Design review of the part built by this model. Coordinates are the model's own, in mm. Round coordinates to 2 decimals unless told otherwise and drop trailing zeros. Loops run counter-clockwise (first coordinate to the right, second up) from the corner with the lowest first, then second, coordinate; pieces in that order, holes last. Notation, with made-up numbers: (67, 76) - (109, 76) arc R23 cw to (109, 97) - close; hole circle Ø9 at (-24, 21). An arc over 180 degrees is marked (long way). Return JSON: item names as keys, results as strings. Group by question number.
(1) Clearance check with a flat-ended pin moving along its axis: pin 1 (12 mm diameter, centred on x = 83, z = 1, fed in from +Y). State where the tip first meets the part, or that it passes through.
(2) The part is to be moulded in two halves that separate along Z. For faces 1 (the cylindrical face through (-82.53, -25.04, 0.84)), 2 (the flat face through (-2, -23, -76.2)), 3 (the flat face through (27, -50.8, 1)), 4 (the cylindrical face through (44.47, -25.04, 0.84)), say which applies: pulls with the +Z half, pulls with the -Z half, needs draft (parallel to the pull), parting line crosses it, or undercut.
(3) We need section A-A, the plane z = 0. Write out the cut boundary in (x, y).
(4) We need section C-C, the plane x = 0. Write out the cut boundary in (y, z).
(5) We need section D-D, the plane x = 60. Write out the cut boundary in (y, z), and give its area (3 significant figures).
(6) Wall thickness on L1, parallel to Z at x = 0, y = -27.5; L2, parallel to Z at x = 106, y = -46; L3, parallel to Z at x = 61.5, y = -4.5: over which ranges is each line inside the solid? List them lowest first. Write a range as [from, to].
(7) We need section B-B, the plane y = -32. Write out the cut boundary in (x, z).
from build123d import *

# Parameters (mm, degrees)
F0_W     = 266.7
F0_H     = 152.4
F1_DEPTH = 50.8
F2_R     = 19.05
F3_DEPTH = 76.2
F4_R     = 19.05
F5_DEPTH = 50.8
F6_R     = 19.05
F7_DEPTH = 50.8
F8_R     = 5.08


with BuildPart() as f1:
    # F0 (on Front) → F1 (new body)
    with BuildSketch(Plane.XZ):
        Rectangle(F0_W, F0_H)
    extrude(amount=F1_DEPTH)

    # F2 (on face) → F3 (cut)
    with BuildSketch(Plane.XZ.offset(50.8)):
        Circle(F2_R)
    extrude(amount=-F3_DEPTH, mode=Mode.SUBTRACT)

    # F4 (on Front) → F5 (cut)
    with BuildSketch(Plane.XZ):
        with Locations((-63.5, 0)):
            Circle(F4_R)
    extrude(amount=F5_DEPTH, mode=Mode.SUBTRACT)

    # F6 (on Front) → F7 (cut)
    with BuildSketch(Plane.XZ):
        with Locations((63.5, 0)):
            Circle(F6_R)
    extrude(amount=F7_DEPTH, mode=Mode.SUBTRACT)

    # F8
    f8_edges = [f1.edges().sort_by_distance(p)[0] for p in [
        (0, -50.8, 76.2),
        (-133.35, -50.8, 0),
        (0, -50.8, -76.2),
        (133.35, -50.8, 0),
    ]]
    fillet(f8_edges, radius=F8_R)


solid = f1.part
Solutions:
{
 "1": {"pin 1": "y = 0"},
 "2": {"face 1": "undercut", "face 2": "pulls with the -Z half", "face 3": "needs draft", "face 4": "undercut"},
 "3": {"outline": "(-133.35, -45.72) arc R5.08 ccw to (-128.27, -50.8) - (-82.55, -50.8) - (-82.55, 0) - (-133.35, 0) - close; (-44.45, -50.8) - (-19.05, -50.8) - (-19.05, 0) - (-44.45, 0) - close; (19.05, -50.8) - (44.45, -50.8) - (44.45, 0) - (19.05, 0) - close; (82.55, -50.8) - (128.27, -50.8) arc R5.08 ccw to (133.35, -45.72) - (133.35, 0) - (82.55, 0) - close"},
 "4": {"outline": "(-50.8, -71.12) arc R5.08 ccw to (-45.72, -76.2) - (0, -76.2) - (0, -19.05) - (-50.8, -19.05) - close; (-50.8, 19.05) - (0, 19.05) - (0, 76.2) - (-45.72, 76.2) arc R5.08 ccw to (-50.8, 71.12) - close"},
 "5": {"outline": "(-50.8, -71.12) arc R5.08 ccw to (-45.72, -76.2) - (0, -76.2) - (0, -18.73) - (-50.8, -18.73) - close; (-50.8, 18.73) - (0, 18.73) - (0, 76.2) - (-45.72, 76.2) arc R5.08 ccw to (-50.8, 71.12) - close", "area": "5,830 mm^2"},
 "6": {"L1": "[-76.2, -19.05], [19.05, 76.2]", "L2": "[-76.19, 76.19]", "L3": "[-76.2, -18.94], [18.94, 76.2]"},
 "7": {"outline": "(-133.35, -76.2) - (133.35, -76.2) - (133.35, 76.2) - (-133.35, 76.2) - close; hole circle Ø38.1 at (-63.5, 0); hole circle Ø38.1 at (0, 0); hole circle Ø38.1 at (63.5, 0)"}
}
